Can you work these out from the model? Positions are in its coordinate system, mm. Face numbers are marked on the shaded views. A direction names the side the tool comes from. Coordinates: 2 decimals unless noted, no trailing zeros. Order: outer loops, then holes, each group sorted by start corner. A loop starts at its lowest first (then second) coordinate and runs counter-clockwise, first axis right, second up. Notation, with made-up numbers: (47.5, 68.5) -> (81.5, 68.5) arc R12 ccw to (81.5, 77.5) -> close; hole circle Ø1 at (47.25, 19.5). An arc over 180 degrees is marked (long way). Write item = value, one per line.
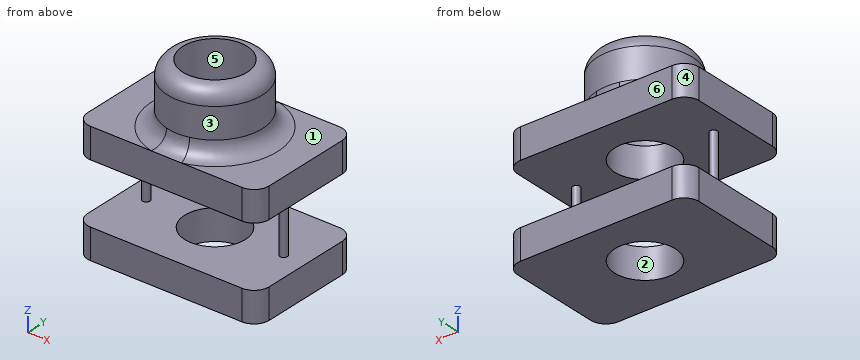
```python
from build123d import *

# Parameters (mm, degrees)
F0_W     = 76.2
F0_H     = 50.8
F0_R     = 12.7
F1_DEPTH = 12.7
F2_R     = 6.35
F3_R     = 1.5875
F4_DEPTH = 25.4
F5_R     = 12.7
F6_DEPTH = 12.7
F7_W     = 6.35
F7_H     = 25.4
F9_R     = 6.34999


# Not quite as in the source:
# - a fillet or chamfer is up to 0.001 mm smaller than in the source, because OpenCascade refuses the exact size


with BuildPart() as f1:
    # F0 (on Top) → F1 (new body)
    with BuildSketch(Plane.XY):
        Rectangle(F0_W, F0_H)
        Circle(F0_R, mode=Mode.SUBTRACT)
    extrude(amount=F1_DEPTH)

    # F2
    f2_edges = [f1.edges().sort_by_distance(p)[0] for p in [
        (38.1, -25.4, 6.35),
        (38.1, 25.4, 6.35),
        (-38.1, -25.4, 6.35),
        (-38.1, 25.4, 6.35),
    ]]
    fillet(f2_edges, radius=F2_R)

    # F3 (on face) → F4 (join)
    with BuildSketch(Plane.XY.offset(12.7)):
        with Locations((-28.8149718722, 0)):
            Circle(F3_R)
        with Locations((28.8149718722, 0)):
            Circle(F3_R)
    extrude(amount=F4_DEPTH)

    # F5 (on face) → F6 (join)
    with BuildSketch(Plane.XY.offset(38.1)):
        with BuildLine():
            Line((-38.1, 19.05), (-38.1, -19.05))
            ThreePointArc((-38.1, -19.05), (-36.2401280605, -23.5401280605), (-31.75, -25.4))
            Line((-31.75, -25.4), (31.75, -25.4))
            ThreePointArc((31.75, -25.4), (36.2401280605, -23.5401280605), (38.1, -19.05))
            Line((38.1, -19.05), (38.1, 19.05))
            ThreePointArc((38.1, 19.05), (36.2401280605, 23.5401280605), (31.75, 25.4))
            Line((31.75, 25.4), (-31.75, 25.4))
            ThreePointArc((-31.75, 25.4), (-36.2401280605, 23.5401280605), (-38.1, 19.05))
        make_face()
        Circle(F5_R, mode=Mode.SUBTRACT)
    extrude(amount=F6_DEPTH)

    # F7 (on Front) → F8 (revolve)
    with BuildSketch(Plane.XZ):
        with Locations((-16.6624, 63.5)):
            Rectangle(F7_W, F7_H)
    revolve(axis=Axis((0, 0, 40.5965745449), (0, 0, 1)))

    # F9 (radius 6.35 in the source; OpenCascade refuses exactly that, so slightly less here)
    f9_edges = [f1.edges().sort_by_distance(p)[0] for p in [
        (19.8374, 0, 76.2),
        (19.8374, 0, 50.8),
    ]]
    fillet(f9_edges, radius=F9_R)


solid = f1.part
```
Item 1: I'm going to push flat-ended pins straight in: P1, Ø8, axis at x = 29, y = -14, coming from the +Z side; P2, Ø1.5, axis at x = 14.5, z = 52.5, coming from the +Y side; P3, Ø9.5, axis at x = 21.5, y = 2.5, coming from the +Z side. Where does each tip first touch, or does it pass through?
A:
P1 = 50.8
P2 = 17.77
P3 = 75.21
Item 2: I want a section at A-A, the plane z = 45.5. Please give me the cut outline in (x, y), plus the area to 3 significant figures.
A:
outline = (-38.1, -19.05) arc R6.35 ccw to (-31.75, -25.4) -> (31.75, -25.4) arc R6.35 ccw to (38.1, -19.05) -> (38.1, 19.05) arc R6.35 ccw to (31.75, 25.4) -> (-31.75, 25.4) arc R6.35 ccw to (-38.1, 19.05) -> close; hole circle Ø25.4 at (0, 0)
area = 3,330 mm2
Item 3: For the marked faces 1, 2 and 3, which set-ups out of +Z, -Z, +X, -X, +Y, -Y let a thin tool reach every point of the face, with its end or its side?
A:
face_1 = +Z, +X
face_2 = +Z, -Z
face_3 = +Z
Item 4: I want a section at B-B, the plane x = 0. Give the number of separate pieces and of enclosed holes in the cut face, plus the area to 3 significant figures.
A:
separate_pieces = 4
enclosed_holes = 0
area = 967 mm2
Item 5: If we mould it in two halves opening along X, with no side actions, what happens to the marked faces 4, 5 and 6? For each: pulls with the +X half, pulls with the -X half, needs draft (parallel to the pull), parting line crosses it, or undercut.
A:
face_4 = pulls with the -X half
face_5 = undercut
face_6 = needs draft
Item 6: If I drill on probe 1 along Z at (x, y) = (21, 17); probe 2 along Y at (x, z) = (0, 5); probe 3 along X at (y, z) = (0, 65.5), over which ranges is the centre line in solid material (lowest first)?
A:
probe_1 = 0 to 12.7, 38.1 to 50.8
probe_2 = -25.4 to -12.7, 12.7 to 25.4
probe_3 = -19.84 to -13.49, 13.49 to 19.84
Item 7: I want a section at C-C, the plane z = 24.5. Please give me the cut outline in (x, y) (1 decimal).
A:
outline = circle Ø3.2 at (-28.8, 0); circle Ø3.2 at (28.8, 0)
